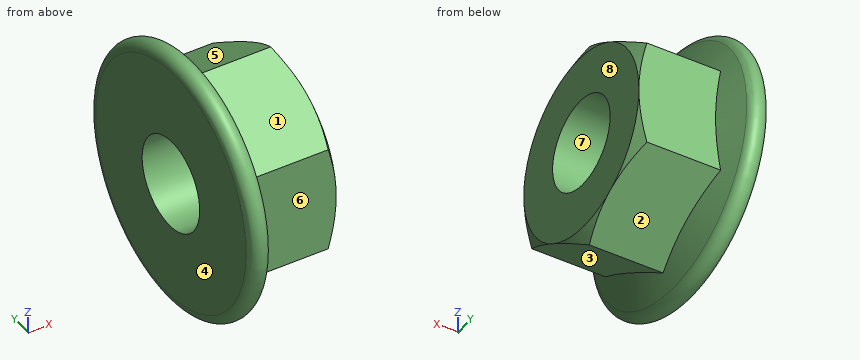
from build123d import *

# Parameters (mm, degrees)
SKETCH1_R      = 2.5
EXTRUDE1_DEPTH = 6


# Read off the part's stored shape, not the designer's step: Cut-Extrude1
with BuildPart() as part:
    # Sketch1 → Extrude1 (new body)
    with BuildSketch(Plane(origin=(0, 0, 0), x_dir=(0, 0, -1), z_dir=(1, 0, 0))):
        Polygon((5.773502692, 0), (2.886751346, 5), (-2.886751346, 5), (-5.773502692, 0), (-2.886751346, -5), (2.886751346, -5), align=None)
        Circle(SKETCH1_R, mode=Mode.SUBTRACT)
    extrude(amount=EXTRUDE1_DEPTH)

    # Cut-Extrude1 outline → Cut-Extrude1 (revolve, cut)
    with BuildSketch(Plane.YX):
        Polygon((5.773502692, 6.000000845), (4.999998834, 6.000000845), (5.773502688, 5.553418015), align=None)
    revolve(axis=Axis((0, 0, 0), (1, 0, 0)), mode=Mode.SUBTRACT)

    # Sketch3 → Revolve1 (revolve)
    with BuildSketch(Plane.XY, mode=Mode.PRIVATE) as revolve1_sk:
        with BuildLine():
            Line((0, 2.5), (0, 6.532899838))
            ThreePointArc((0, 6.532899838), (0.468624253, 7.091384474), (1.1, 6.726859517))
            Line((1.1, 6.726859517), (2.638451048, 2.5))
            Line((2.638451048, 2.5), (0, 2.5))
        make_face()
    revolve(revolve1_sk.sketch.rotate(Axis((0, 0, 0), (1, 0, 0)), 90), axis=Axis((0, 0, 0), (1, 0, 0)))


solid = part.part
Could you check a few things on this model? Use its own coordinates, in mm. Face numbers are marked on the shaded views. A direction names the side the tool comes from. Give positions to 0.01 mm unless a question says otherwise; leave off trailing zeros. Return JSON: item names as keys, results as strings.
Item 1: Which directions (+Z, -Z, +X, -X, +Y, -Y) give clear straight access to the entire face, cutting with the end or side of a thin tool? Please do the marked faces 1, 2, 3 and 4.
Geometry results:
{"face 1": "+Z, +X, -Y", "face 2": "-Z, +X, +Y", "face 3": "-Z, +X, -Y", "face 4": "+Z, -Z, -X, +Y, -Y"}
Item 2: We'd pull the mould along Y, two halves only. Please class the marked faces 5, 6, 7 and 8: +Y half, -Y half, draft (parallel to the pull), parting line (faces both ways), or undercut.
Geometry results:
{"face 5": "+Y half", "face 6": "-Y half", "face 7": "undercut", "face 8": "draft"}
Item 3: I need wall thicknesses on L1, parallel to Y at x = 4.85, z = 0; L2, parallel to Y at x = 5.5, z = -1.25; L3, parallel to Z at x = 0.75, y = -2. Which ranges of each line are inside material? Lowest first, please. Write a range as from..to.
Geometry results:
{"L1": "y = -5..-2.5, 2.5..5", "L2": "y = -5..-2.17, 2.17..5", "L3": "z = -6.78..-1.5, 1.5..6.78"}
Item 4: I'm going to push flat-ended pins straight in: pin 1 (1.4 mm diameter, centred on x = 3.5, z = 0.5, fed in from -Y); pin 2 (1 mm diameter, centred on x = 4, y = -2, fed in from +Z); pin 3 (1 mm diameter, centred on y = -5, z = 5, fed in from +X). Where does each tip first touch, or does it pass through?
Geometry results:
{"pin 1": "stops at y = -5", "pin 2": "stops at z = 4.91", "pin 3": "stops at x = 1.16"}
